Geometry check sheet. Reference: the model listing, model coordinates, mm. Face numbers are marked on the shaded views. A direction names the side the tool comes from. Coordinates: 2 decimals unless noted, no trailing zeros. Order: outer loops, then holes, each group sorted by start corner. A loop starts at its lowest first (then second) coordinate and runs counter-clockwise, first axis right, second up. Notation, with made-up numbers: (9, -1) - (32, -1) arc R29 ccw to (32, 32) - close; hole circle Ø9 at (36, -40). An arc over 180 degrees is marked (long way). Put each result on its own line as item: value.
from build123d import *

# Parameters (mm, degrees)
BOSS_EXTRUDE1_DEPTH    = 69.36
CONVERT_SOLID2_DEPTH   = 69.36
CONVERT_SOLID2_2_DEPTH = 69.36
CUT_EXTRUDE1_DEPTH     = 78.896254724


# Read off the part's stored shape, not the designer's step: Convert-Solid2
with BuildPart() as part:
    # Sketch2 → Boss-Extrude1 (new body)
    with BuildSketch(Plane(origin=(0, 0, 0), x_dir=(1, 0, 0), z_dir=(0, 1, 0))):
        Polygon((0, 11.95), (0, 0), (34.05, 0), (34.05, 11.95), (31.98, 11.95), (31.98, 2.07), (2.07, 2.07), (2.07, 11.95), align=None)
    extrude(amount=BOSS_EXTRUDE1_DEPTH)

    # Convert-Solid2 outline → Convert-Solid2 (cut)
    with BuildSketch(Plane(origin=(0, 0, 0), x_dir=(1, 0, 0), z_dir=(0, 1, 0))):
        with BuildLine():
            ThreePointArc((34.05, 4.450000066), (32.746625157, 1.303374843), (29.599999934, 0))
            Line((29.599999934, 0), (34.05, 0))
            Line((34.05, 0), (34.05, 4.450000066))
        make_face()
        with BuildLine():
            Line((0, 0), (4.450000066, 0))
            ThreePointArc((4.450000066, 0), (1.303374843, 1.303374843), (0, 4.450000066))
            Line((0, 4.450000066), (0, 0))
        make_face()
    extrude(amount=CONVERT_SOLID2_DEPTH, mode=Mode.SUBTRACT)

    # Convert-Solid2 2 outline → Convert-Solid2 2 (add)
    with BuildSketch(Plane(origin=(0, 0, 0), x_dir=(1, 0, 0), z_dir=(0, 1, 0))):
        with BuildLine():
            Line((2.07, 2.07), (4.450000066, 2.07))
            ThreePointArc((4.450000066, 2.07), (2.76708588, 2.76708588), (2.07, 4.450000066))
            Line((2.07, 4.450000066), (2.07, 2.07))
        make_face()
        with BuildLine():
            ThreePointArc((31.98, 4.450000066), (31.28291412, 2.76708588), (29.599999934, 2.07))
            Line((29.599999934, 2.07), (31.98, 2.07))
            Line((31.98, 2.07), (31.98, 4.450000066))
        make_face()
    extrude(amount=CONVERT_SOLID2_2_DEPTH)

    # Sketch12 → Cut-Extrude1 (cut, through all)
    with BuildSketch(Plane(origin=(0, 0, -2.07), x_dir=(-1, 0, 0), z_dir=(0, 0, -1))):
        with BuildLine():
            Line((-21.46, 18.18), (-21.46, 51.18))
            ThreePointArc((-21.46, 51.18), (-17.025, 55.615), (-12.59, 51.18))
            Line((-12.59, 51.18), (-12.59, 18.18))
            ThreePointArc((-12.59, 18.18), (-17.025, 13.745), (-21.46, 18.18))
        make_face()
    extrude(amount=-CUT_EXTRUDE1_DEPTH, mode=Mode.SUBTRACT)


solid = part.part
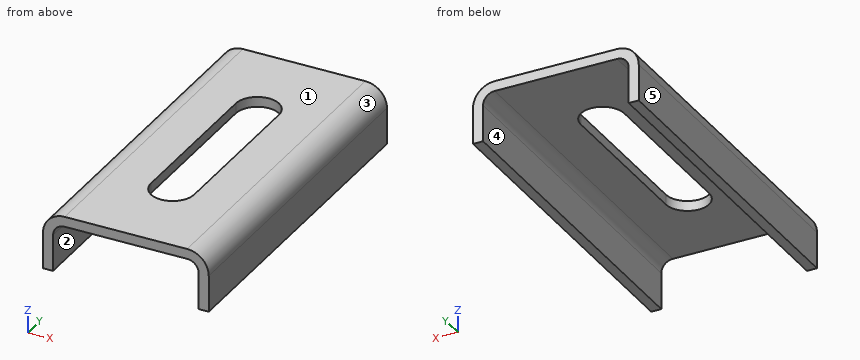
Q1. Section check D-D on x = 7. Record the boundary of the cut face in (y, z).
Answer block:
outline: (0, -2.07) - (69.36, -2.07) - (69.36, 0) - (0, 0) - close
Q2. Section check B-B on y = 48.5. Record the boundary of the cut face in (x, z), then the cut area to 3 significant figures.
Answer block:
outline: (0, -11.95) - (2.07, -11.95) - (2.07, -4.45) arc R2.38 cw to (4.45, -2.07) - (12.59, -2.07) - (12.59, 0) - (4.45, 0) arc R4.45 ccw to (0, -4.45) - close; (21.46, -2.07) - (29.6, -2.07) arc R2.38 cw to (31.98, -4.45) - (31.98, -11.95) - (34.05, -11.95) - (34.05, -4.45) arc R4.45 ccw to (29.6, 0) - (21.46, 0) - close
area: 87.0 mm^2
Q3. Thickness scan on L1, parallel to X at y = 51.5, z = -8.5; L2, parallel to Z at x = 18.5, y = 6.5; L3, parallel to X at y = 16.5, z = -2.5. Record the ranges inside material, lowest first. Write a range as [from, to].
Answer block:
L1: x = [0, 2.07], [31.98, 34.05]
L2: z = [-2.07, 0]
L3: x = [0.45, 3.09], [30.96, 33.6]
Q4. Section check A-A on z = -6.25. Record the boundary of the cut face in (x, y).
Answer block:
outline: (0, 0) - (2.07, 0) - (2.07, 69.36) - (0, 69.36) - close; (31.98, 0) - (34.05, 0) - (34.05, 69.36) - (31.98, 69.36) - close
Q5. Access from +Z, -Z, +X, -X, +Y, -Y to the whole of each face (thin tool, end or side, straight path). Record for the marked faces 1 and 2.
Answer block:
face 1: +Z, +X, -X, +Y, -Y
face 2: -Z, +Y, -Y
Q6. Depth check by flat-ended pin: pin 1 Ø1 at (y, z) = (38, -0.5) entering from -X; pin 2 Ø5 at (y, z) = (16.5, -1.5) entering from -X; pin 3 Ø20 at (x, y) = (14, 48.5) entering from -Z. Enter the tip coordinate at first touch or a pass-through.
Answer block:
pin 1: stops at x = 1.64
pin 2: stops at x = 0.02
pin 3: stops at z = -2.11
Q7. Draft check along X on the marked faces 3, 4 and 5. Enter one of: pulls with the +X half, pulls with the -X half, needs draft (parallel to the pull), parting line crosses it, or undercut.
Answer block:
face 3: pulls with the +X half
face 4: undercut
face 5: pulls with the -X half
Q8. Section check C-C on x = 14.5. Record the boundary of the cut face in (y, z), then the cut area to 3 significant figures.
Answer block:
outline: (0, -2.07) - (14.53, -2.07) - (14.53, 0) - (0, 0) - close; (54.83, -2.07) - (69.36, -2.07) - (69.36, 0) - (54.83, 0) - close
area: 60.2 mm^2
